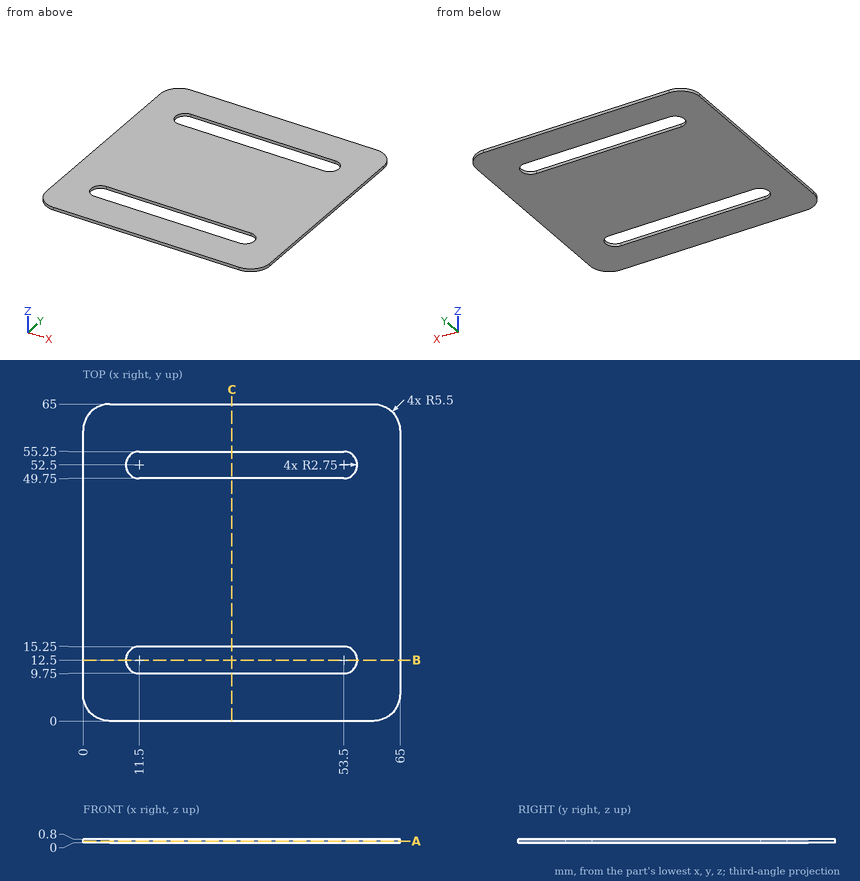
Geometry: see drawing. Coordinates: mm, zero at the bounding-box minimum. Coordinates: 2 decimals unless noted, no trailing zeros. Loops run counter-clockwise (first coordinate to the right, second up) from the corner with the lowest first, then second, coordinate; pieces in that order, holes last. Notation, with made-up numbers: (60.5, -20.5) - (89.5, -20.5) arc R13 cw to (89.5, -14.5) - close; hole circle Ø2 at (64.25, -7). An arc over 180 degrees is marked (long way). Put each result on its own line as item: value. Start each with the question number.
Q1. Cut plane C-C, the plane x = 30.5. Return loops of the section in (y, z).
Q2. Cut plane A-A, the plane z = 0.35. Return loops of the section in (x, y), and give its area (3 significant figures).
Q3. Line query: line 1 (Y direction, x = 45, z = 0.2); line 2 (X direction, y = 54.5, z = 0.6); line 3 (X direction, y = 53.5, z = 0.4). Output: solid intervals per line, ascending.
Q4. Cut plane B-B, the plane y = 12.5. Return loops of the section in (x, z).
Filled sheet:
1. outline: (0, 0) - (9.75, 0) - (9.75, 0.8) - (0, 0.8) - close; (15.25, 0) - (49.75, 0) - (49.75, 0.8) - (15.25, 0.8) - close; (55.25, 0) - (65, 0) - (65, 0.8) - (55.25, 0.8) - close
2. outline: (0, 5.5) arc R5.5 ccw to (5.5, 0) - (59.5, 0) arc R5.5 ccw to (65, 5.5) - (65, 59.5) arc R5.5 ccw to (59.5, 65) - (5.5, 65) arc R5.5 ccw to (0, 59.5) - close; hole (11.5, 9.75) - (53.5, 9.75) arc R2.75 ccw to (53.5, 15.25) - (11.5, 15.25) arc R2.75 ccw to start; hole (11.5, 49.75) - (53.5, 49.75) arc R2.75 ccw to (53.5, 55.25) - (11.5, 55.25) arc R2.75 ccw to start
2. area: 3,690 mm²
3. line 1: 0 to 9.75, 15.25 to 49.75, 55.25 to 65
3. line 2: 0 to 9.61, 55.39 to 65
3. line 3: 0 to 8.94, 56.06 to 65
4. outline: (0, 0) - (8.75, 0) - (8.75, 0.8) - (0, 0.8) - close; (56.25, 0) - (65, 0) - (65, 0.8) - (56.25, 0.8) - close
